```python
from build123d import *

# Parameters (mm, degrees)
TAP_DRILL_FOR_M3X0_5_TAP1_D     = 2.5
TAP_DRILL_FOR_M3X0_5_TAP1_DEPTH = 6
TAP_DRILL_FOR_M3X0_5_TAP1_TIP   = 0.751075774
TAP_DRILL_FOR_M3X0_5_TAP2_D     = 2.5
TAP_DRILL_FOR_M3X0_5_TAP2_DEPTH = 6
TAP_DRILL_FOR_M3X0_5_TAP2_TIP   = 0.751075774


with BuildPart() as part:
    # Sketch1 → Revolve1 (revolve)
    with BuildSketch(Plane.XY, mode=Mode.PRIVATE) as revolve1_sk:
        Polygon((0, 0), (0, 33.5), (-21.5, 33.5), (-45, 29.6), (-45, 14.1), (-43, 14.1), (-43, 12.6), (-45, 12.6), (-45, 8.3), (-26.5, 5.6), (-26.5, 0), align=None)
    revolve(revolve1_sk.sketch.rotate(Axis((0, 0, 0), (0, -1, 0)), 270), axis=Axis((0, 0, 0), (0, -1, 0)))

    # Tap Drill for M3x0.5 Tap1
    with Locations(Plane(origin=(0, 33.5, 0), x_dir=(1, 0, 0), z_dir=(0, 1, 0))):
        with Locations((0, 17.5), (12.374368671, 12.374368671), (17.5, 0), (12.374368671, -12.374368671), (0, -17.5), (-12.374368671, -12.374368671), (-17.5, 0), (-12.374368671, 12.374368671), (0, 0)):
            Hole(TAP_DRILL_FOR_M3X0_5_TAP1_D / 2, depth=TAP_DRILL_FOR_M3X0_5_TAP1_DEPTH)
            with Locations((0, 0, -(TAP_DRILL_FOR_M3X0_5_TAP1_DEPTH + TAP_DRILL_FOR_M3X0_5_TAP1_TIP / 2))):  # 118° drill point
                Cone(0, TAP_DRILL_FOR_M3X0_5_TAP1_D / 2, TAP_DRILL_FOR_M3X0_5_TAP1_TIP, mode=Mode.SUBTRACT)

    # Tap Drill for M3x0.5 Tap2
    with Locations(Plane(origin=(0, 0, 0), x_dir=(-1, 0, 0), z_dir=(0, -1, 0))):
        with Locations((0, 15), (15, 0), (0, -15), (-15, 0), (0, 0)):
            Hole(TAP_DRILL_FOR_M3X0_5_TAP2_D / 2, depth=TAP_DRILL_FOR_M3X0_5_TAP2_DEPTH)
            with Locations((0, 0, -(TAP_DRILL_FOR_M3X0_5_TAP2_DEPTH + TAP_DRILL_FOR_M3X0_5_TAP2_TIP / 2))):  # 118° drill point
                Cone(0, TAP_DRILL_FOR_M3X0_5_TAP2_D / 2, TAP_DRILL_FOR_M3X0_5_TAP2_TIP, mode=Mode.SUBTRACT)


solid = part.part
```
Check sheet for the modelled part. Datum: model origin and axes. Units: mm. A direction names the side the tool comes from. Give positions to 0.01 mm unless a question says otherwise; leave off trailing zeros. Order: outer loops, then holes, each group sorted by start corner. A loop starts at its lowest first (then second) coordinate and runs counter-clockwise, first axis right, second up. Notation, with made-up numbers: M -16,41.5 L -5,41.5 A17 ccw -5,48.5 Z; hole C 2,-8 d9. An arc over 180 degrees is marked long. Answer in a Markdown table with one row per item. Add a question column.
Q1. Access from +Z, -Z, +X, -X, +Y, -Y to the whole of each face (thin tool, end or side, straight path). Record for faces 1 (the cylindrical face through (-18.655, 30.458, 0.479)), 2 (the cylindrical face through (0.672, 3.042, -16.054)), 3 (the flat face through (36.5, 14.1, 23.1)).
Q2. Thickness scan on L1, parallel to Y at x = -31, z = 3; L2, parallel to Y at x = 1, z = -27.5; L3, parallel to Z at x = -17, y = 29. Record the ranges inside material, lowest first.
Q3. Sectioned sample at A-A, the plane y = 9.5. Record the boundary of the cut face in (x, z).
Q4. Release check for a two-part mould opening along Y. For faces 4 (the conical face through (17.7, 26.88, 0.08)), 5 (the flat face through (0, 0, 6)), 6 (the cylindrical face through (-29.061, 13.34, -31.693)), 7 (the cylindrical face through (-26.274, 2.761, -3.45)) record: released by +Y, released by -Y, zero draft, split by the parting line, or undercut.
Q5. Gauge pin test, flat ends, axial feed: pin 1 Ø1.5 at (x, z) = (12.37, 12.37) entering from -Y; pin 2 Ø4 at (y, z) = (22, 4.5) entering from -X; pin 3 Ø1 at (x, y) = (-22.5, 14.5) entering from -Z; pin 4 Ø2 at (x, z) = (-15, 0) entering from -Y. Record the tip position at first contact, or that the pin passes through.
Verdict:
| question | item | result |
|---|---|---|
| 1 | face 1 | +Y |
| 1 | face 2 | -Y |
| 1 | face 3 | none |
| 2 | L1 | 6.28 to 31.9 |
| 2 | L2 | 5.75 to 32.5 |
| 2 | L3 | -41.67 to -1.15, 1.15 to 41.67 |
| 3 | outline | C 0,0 d90 |
| 4 | face 4 | released by +Y |
| 4 | face 5 | released by -Y |
| 4 | face 6 | undercut |
| 4 | face 7 | zero draft |
| 5 | pin 1 | y = 0 |
| 5 | pin 2 | x = -44.93 |
| 5 | pin 3 | z = -39.26 |
| 5 | pin 4 | y = 6.15 |
